Study the drawing (mm; zero at the part's minimum x, y, z) and answer. Coordinates: 2 decimals unless noted, no trailing zeros. Write each loop counter-clockwise with the first axis right and the second up, starting at its lowest first coordinate (ties: lowest second). Pieces come first, ordered by that corner, then holes. Notation, with made-up numbers: (69, 39.25) - (95, 39.25) arc R13 ccw to (95, 45.25) - close; hole circle Ø1 at (55, 31). An arc over 180 degrees is marked (long way). One line per item, written item: value.
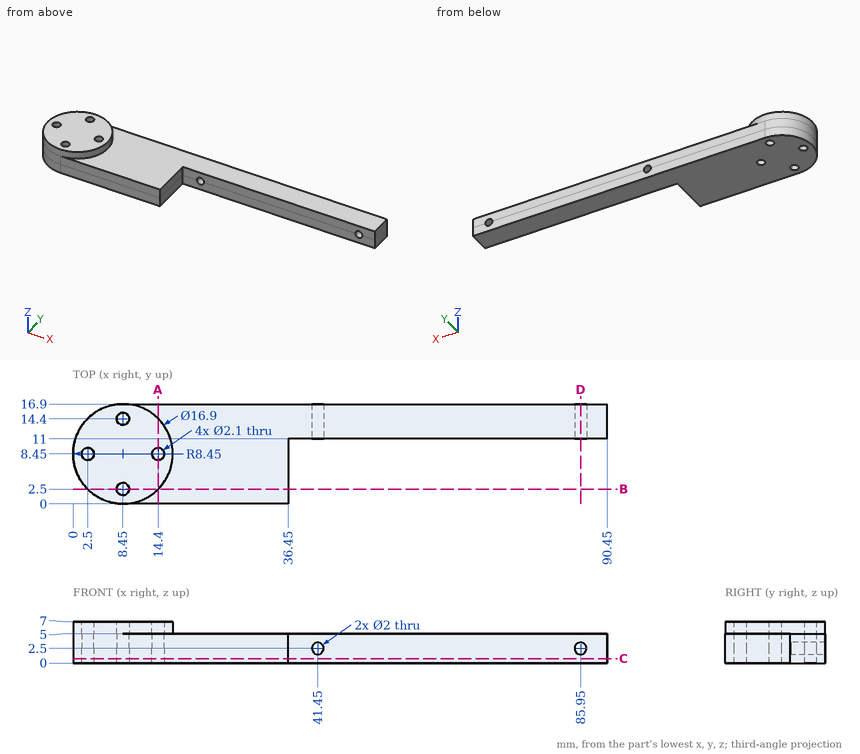
Item 1: Given pin 1 (1.5 mm diameter, centred on y = 3.5, z = 2, fed in from -X); pin 2 (4 mm diameter, centred on y = 2.5, z = 2, fed in from -X); pin 3 (1.7 mm diameter, centred on x = 2.5, y = 8.45, fed in from -Z); pin 4 (2 mm diameter, centred on x = 62, z = 2, fed in from -Y), each flat-ended and moving along its own axis, determine where each tip first touches the part or whether it passes through.
Evaluation:
pin 1: stops at x = 1.12
pin 2: stops at x = 0.98
pin 3: passes through
pin 4: stops at y = 11
Item 2: Section C-C, the plane z = 0.75 is taken. Determine the outline of the cut face in (x, y), then the cut area to 3 significant figures.
Evaluation:
outline: (8.45, 0) - (36.45, 0) - (36.45, 11) - (90.45, 11) - (90.45, 16.9) - (8.45, 16.9) arc R8.45 ccw to start; hole circle Ø2.1 at (2.5, 8.45); hole circle Ø2.1 at (8.45, 2.5); hole circle Ø2.1 at (8.45, 14.4); hole circle Ø2.1 at (14.4, 8.45)
area: 890 mm2
Item 3: Section A-A, the plane x = 14.4 is taken. Determine the outline of the cut face in (y, z).
Evaluation:
outline: (0, 0) - (7.4, 0) - (7.4, 7) - (2.45, 7) - (2.45, 5) - (0, 5) - close; (9.5, 0) - (16.9, 0) - (16.9, 5) - (14.45, 5) - (14.45, 7) - (9.5, 7) - close
Item 4: Section B-B, the plane y = 2.5 is taken. Determine the outline of the cut face in (x, z).
Evaluation:
outline: (2.45, 0) - (7.4, 0) - (7.4, 7) - (2.45, 7) - close; (9.5, 0) - (36.45, 0) - (36.45, 5) - (14.45, 5) - (14.45, 7) - (9.5, 7) - close
Item 5: Consider probe 1 along X at (y, z) = (8.45, 3.55); probe 2 along Y at (x, z) = (8.45, 1). Determine where each line is inside the solid, lowest interval first.
Evaluation:
probe 1: x = 0 to 1.45, 3.55 to 13.35, 15.45 to 36.45
probe 2: y = 0 to 1.45, 3.55 to 13.35, 15.45 to 16.9
Item 6: Section D-D, the plane x = 85.95 is taken. Determine the outline of the cut face in (y, z).
Evaluation:
outline: (11, 0) - (16.9, 0) - (16.9, 1.5) - (11, 1.5) - close; (11, 3.5) - (16.9, 3.5) - (16.9, 5) - (11, 5) - close
